Autodesk Inventor part; units mm, degrees
ref_plane "YZ Plane" through (0, 0, 0) normal (1, 0, 0) x (0, 1, 0)
ref_plane "XZ Plane" through (0, 0, 0) normal (0, 1, 0) x (-1, 0, 0)
ref_plane "XY Plane" through (0, 0, 0) normal (0, 0, 1) x (1, 0, 0)
sketch "Sketch1" plane through (0, 0, 0) normal (0, 1, 0) x (-1, 0, 0)
  line L0 (0, 0) -> (70, 0)
  line L1 (70, 0) -> (70, -30)
  line L2 (70, -30) -> (0, -30)
  line L3 (0, -30) -> (0, 0)
  dimension "d0" = 70
  dimension "d1" = 30
extrude "Extrusion1" add sketch "Sketch1" along normal blind 20
fillet "Fillet1" radius 2 11 edges at (-70, 10, 0) (-70, 20, -15) (-35, 20, 0) (-70, 0, -15) (-35, 0, 0) (0, 10, 0) (0, 20, -15) (0, 0, -15) (0, 10, -30) (-35, 20, -30) (-35, 0, -30)
sketch "Sketch2" plane through (0, 20, 0) normal (0, 1, 0) x (1, 0, 0)
  line L0 (-67.0416, 18.9322) -> (-64.0416, 18.9322)
  line L1 (-64.0416, 18.9322) -> (-64.0416, 24.9322)
  line L2 (-64.0416, 24.9322) -> (-67.0416, 24.9322)
  line L3 (-67.0416, 24.9322) -> (-67.0416, 18.9322)
  point P0 (0, 0)
  dimension "d6" = 3
  dimension "d7" = 6
fillet "Fillet2" radius 2 3 edges at (-69.4142, 19.4142, -29.4142) (-69.4142, 0.5858, -29.4142) (-70, 10, -30)
extrude "Extrusion2" cut sketch "Sketch2" against normal blind 4
sketch "Sketch3" plane through (0, 16, 0) normal (0, 1, 0) x (1, 0, 0)
  line L0 (-64.0416, 18.9322) -> (-67.0416, 18.9322)
  line L1 (-67.0416, 18.9322) -> (-67.0416, 24.9322)
  line L2 (-64.0416, 18.9322) -> (-67.0416, 18.9322)
  line L3 (-67.0416, 18.9322) -> (-67.0416, 21.9322)
  line L4 (-67.0416, 21.9322) -> (-64.0416, 21.9322)
  line L5 (-64.0416, 21.9322) -> (-64.0416, 18.9322)
  point P0 (0, 0)
extrude "Extrusion3" add sketch "Sketch3" along normal blind 8
equation "\"BendRadius\" = Thickness"
equation "\"BendReliefWidth\" = Thickness"
equation "\"BendReliefDepth\" = 0.5 * Thickness"
equation "\"CornerReliefSize\" = 4 * Thickness"
equation "\"MinimumRemnant\" = 2 * Thickness"
equation "\"TransitionRadius\" = BendRadius"
equation "\"JacobiRadiusSize\" = BendRadius"
equation "\"GapSize\" = Thickness"
Build history of the part. All positions in model axes, mm. A direction names the side the tool comes from. Coordinates: 2 decimals unless noted, no trailing zeros. Write each loop counter-clockwise with the first axis right and the second up, starting at its lowest first coordinate (ties: lowest second). Pieces come first, ordered by that corner, then holes.
1. Band-saw the part on B-B, the plane x = -27.5. Give the cut face in (y, z), and give its area (3 significant figures).
Answer block:
outline: (0, -28) arc R2 ccw to (2, -30) - (18, -30) arc R2 ccw to (20, -28) - (20, -2) arc R2 ccw to (18, 0) - (2, 0) arc R2 ccw to (0, -2) - close
area: 597 mm2
2. 3-axis set-ups, long thin cutter, end or side, ignore diameter. For faces 4 (the flat face through (-67.042, 18, -23)), 5 (the flat face through (-66, 22, -18.932)), 6 (the flat face through (-64.042, 22, -20)): which of +Z, -Z, +X, -X, +Y, -Y reach the whole face in a straight line?
Answer block:
face 4: +Y
face 5: +Z, +X, -X, +Y
face 6: +Z, -Z, +X, +Y
3. Band-saw the part on D-D, the plane z = -16. Give the cut face in (x, y), and give its area (3 significant figures).
Answer block:
outline: (-70, 2) arc R2 ccw to (-68, 0) - (-2, 0) arc R2 ccw to (0, 2) - (0, 18) arc R2 ccw to (-2, 20) - (-68, 20) arc R2 ccw to (-70, 18) - close
area: 1,400 mm2
4. Drill centre lines: probe 1 along Y at (x, z) = (-37, -3.75); probe 2 along X at (y, z) = (8.25, -1.5). Where is each one in solid material? Low to high.
Answer block:
probe 1: y = 0 to 20
probe 2: x = -69.94 to -0.06
5. Pull direction X, two halves, no side cores. Call faces 1 (the cylindrical face through (-69.43, 9.89, -29.4)), 2 (the cylindrical face through (-34.54, 19.4, -29.43)), 3 (the flat face through (-66, 18, -24.932)): released by +X, released by -X, zero draft, split by the parting line, or undercut.
Answer block:
face 1: released by -X
face 2: zero draft
face 3: undercut
6. Band-saw the part on A-A, the plane z = -20.75. Give the cut face in (x, y).
Answer block:
outline: (-70, 2) arc R2 ccw to (-68, 0) - (-2, 0) arc R2 ccw to (0, 2) - (0, 18) arc R2 ccw to (-2, 20) - (-64.04, 20) - (-64.04, 24) - (-67.04, 24) - (-67.04, 20) - (-68, 20) arc R2 ccw to (-70, 18) - close
7. Band-saw the part on C-C, the plane y = 22.5. Give the cut face in (x, z), and give its area (3 significant figures).
Answer block:
outline: (-67.04, -21.93) - (-64.04, -21.93) - (-64.04, -18.93) - (-67.04, -18.93) - close
area: 9.00 mm2
8. Drop flat-ended pins along their axis: pin 1 (1.5 mm diameter, centred on y = 21, z = -20.5, fed in from -X); pin 2 (1.5 mm diameter, centred on y = 20.5, z = -14.5, fed in from -X); pin 3 (6 mm diameter, centred on x = -62.5, z = -12.5, fed in from +Y). Give the stop position or say it passes through.
Answer block:
pin 1: stops at x = -67.04
pin 2: stops at x = -68.97
pin 3: stops at y = 20
